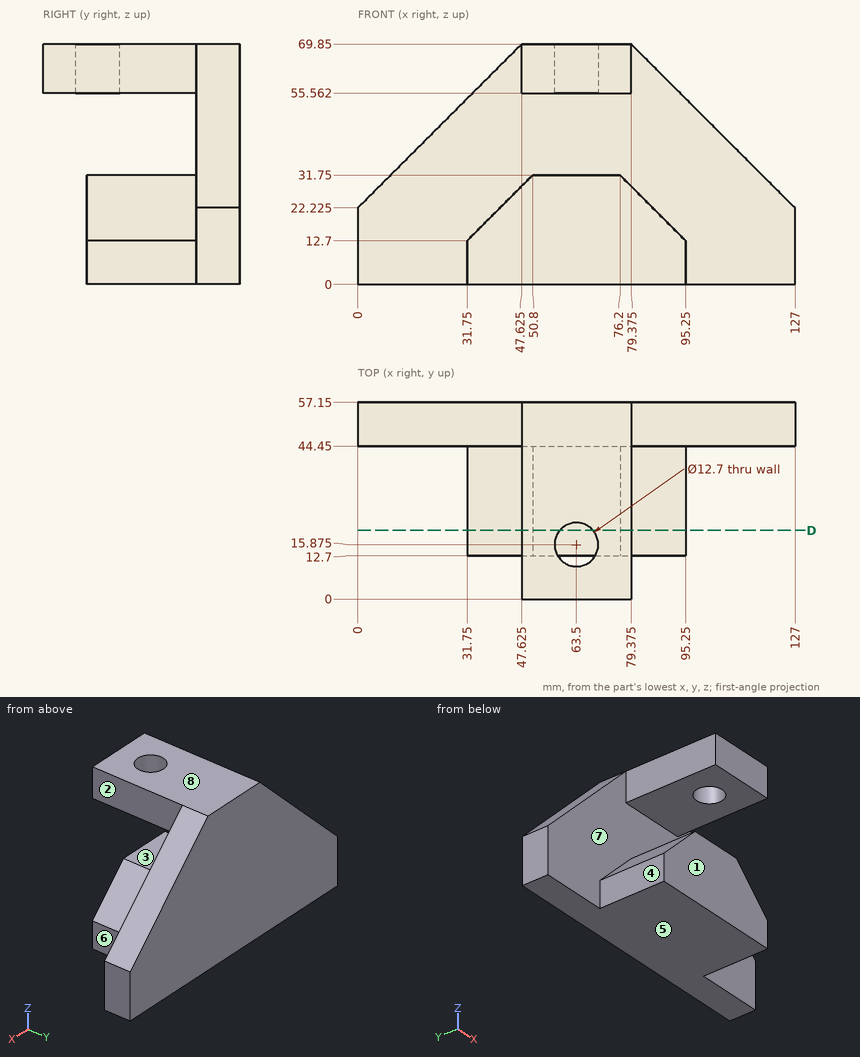
Design review of the part shown in the three views and the two pictorial views. Dimensions are in mm from the part's minimum x, y and z. A direction names the side the tool comes from. Round coordinates to 2 decimals unless told otherwise and drop trailing zeros.
1) The part is to be moulded in two halves that separate along Z. For the marked faces 5, 6, 7 and 8, say which applies: pulls with the +Z half, pulls with the -Z half, needs draft (parallel to the pull), parting line crosses it, or undercut.
Values follow:
face 5: pulls with the -Z half
face 6: needs draft
face 7: undercut
face 8: pulls with the +Z half
2) Clearance check with flat-ended pins moving along their axes: P1, Ø12, axis at y = 36, z = 55, coming from the +X side (1 decimal); P2, Ø1.5, axis at y = 48, z = 47, coming from the +X side (1 decimal); P3, Ø12, axis at y = 10.5, z = 35, coming from the -X side. State where each tip first meets the part, or that it passes through.
Values follow:
P1: stops at x = 79.4
P2: stops at x = 103
P3: stops at x = 48.47
3) Wall thickness on line 1 along Z through (x, y) = (60, 44); line 2 along Z through (x, y) = (58, 8); line 3 along Y through (x, z) = (53, 13.5): over which ranges is each line inside the solid? List them lowest first.
Values follow:
line 1: z = 0 to 31.75, 55.56 to 69.85
line 2: z = 55.56 to 69.85
line 3: y = 12.7 to 57.15
4) Tool access review of the marked faces 1, 2, 3 and 4: name each direction out of +Z, -Z, +X, -X, +Y, -Y from which nothing blocks a thin tool from reaching the whole face with its end or side.
Values follow:
face 1: -Z, +X, -X, -Y
face 2: +Z, +X, -Y
face 3: +X, -X, -Y
face 4: +Z, -Z, -X, -Y
5) Consider section D-D on y = 20. Give the number of separate pieces and of enclosed holes in the cut face, then the cut area to 3 significant figures.
Values follow:
separate pieces: 3
enclosed holes: 0
area: 1,970 mm2
